CAD build for the part. Positions are in the model's coordinates, mm. Give positions to 0.01 mm unless a question says otherwise; leave off trailing zeros. Loops run counter-clockwise (first coordinate to the right, second up) from the corner with the lowest first, then second, coordinate; pieces in that order, holes last. Notation, with made-up numbers: (69, -22.5) - (81, -22.5) arc R26 cw to (81, 1.5) - close; hole circle Ø6 at (86, 18.25). An arc over 180 degrees is marked (long way). Return JSON: item names as keys, results as strings.
from build123d import *

# Parameters (mm, degrees)
F1_DEPTH    = 25
F1_FACE_R   = 24.15
F1_FACE_R_2 = 20.15
F2_DEPTH    = 50
F2_FACE_R   = 24.15
F2_FACE_R_2 = 20.15
F3_DEPTH    = 1000


with BuildPart() as f1:
    # F0 (on Front) → F1 (new body)
    with BuildSketch(Plane.XZ):
        with BuildLine():
            ThreePointArc((0, -24.15), (17.076629, -17.076629), (24.15, 0))
            ThreePointArc((24.15, 0), (-17.076629, 17.076629), (0, -24.15))
        make_face()
        with BuildLine():
            ThreePointArc((20.15, 0), (14.248202, -14.248202), (0, -20.15))
            ThreePointArc((0, -20.15), (-14.248202, 14.248202), (20.15, 0))
        make_face(mode=Mode.SUBTRACT)
    extrude(amount=F1_DEPTH)

    # F1_face (on face) → F2 (join)
    with BuildSketch(Plane(origin=(0, 0, 0), x_dir=(1, 0, 0), z_dir=(0, 1, 0))):
        Circle(F1_FACE_R)
        Circle(F1_FACE_R_2, mode=Mode.SUBTRACT)
    extrude(amount=F2_DEPTH)

    # F2_face (on face) → F3 (join)
    with BuildSketch(Plane(origin=(0, 50, 0), x_dir=(1, 0, 0), z_dir=(0, 1, 0))):
        Circle(F2_FACE_R)
        Circle(F2_FACE_R_2, mode=Mode.SUBTRACT)
    extrude(amount=F3_DEPTH)


solid = f1.part
1. Cut at B-B, the plane x = 12. Write the cut outline in (y, z), plus the area to 3 significant figures.
Values follow:
{"outline": "(-25, -20.96) - (1050, -20.96) - (1050, -16.19) - (-25, -16.19) - close; (-25, 16.19) - (1050, 16.19) - (1050, 20.96) - (-25, 20.96) - close", "area": "10,300 mm²"}
2. Cut at C-C, the plane y = 983. Write the cut outline in (x, z).
Values follow:
{"outline": "circle Ø48.3 at (0, 0); hole circle Ø40.3 at (0, 0)"}
3. Drop flat-ended pins along their axis: P1, Ø2, axis at x = -12.5, y = 872, coming from the -Z side; P2, Ø4, axis at x = 12.5, y = 427.5, coming from the +Z side; P3, Ø1.5, axis at x = 7, y = 108, coming from the +Z side. Give the stop position or say it passes through.
Values follow:
{"P1": "stops at z = -21.24", "P2": "stops at z = 21.75", "P3": "stops at z = 23.33"}
4. Drill centre lines: probe 1 along Z at (x, y) = (0, 342); probe 2 along X at (y, z) = (216, -1.5); probe 3 along Z at (x, y) = (-17, 618). Where is each one in solid material? Low to high.
Values follow:
{"probe 1": "z = -24.15 to -20.15, 20.15 to 24.15", "probe 2": "x = -24.1 to -20.09, 20.09 to 24.1", "probe 3": "z = -17.15 to -10.82, 10.82 to 17.15"}
5. Cut at A-A, the plane z = -12. Write the cut outline in (x, y).
Values follow:
{"outline": "(-20.96, -25) - (-16.19, -25) - (-16.19, 1050) - (-20.96, 1050) - close; (16.19, -25) - (20.96, -25) - (20.96, 1050) - (16.19, 1050) - close"}
